Job drawing, mm, ordinate dimensions from the low corner. One solid piece. A direction names the side the tool comes from. Round coordinates to 2 decimals unless told otherwise and drop trailing zeros. Write each loop counter-clockwise with the first axis right and the second up, starting at its lowest first coordinate (ties: lowest second). Pieces come first, ordered by that corner, then holes.
1) Pull direction X, two halves, no side cores. Call the marked faces 1, 2 and 3: +X half, -X half, draft (parallel to the pull), parting line (faces both ways), or undercut.
2) Saw through at B-B (z = 15.5). Write the cut outline in (x, y).
3) Flat gauge pins, fed straight in: pin 1 (2 mm diameter, centred on y = 10, z = 14.5, fed in from +X); pin 2 (6.5 mm diameter, centred on x = 84, y = 5, fed in from -Z); pin 3 (5 mm diameter, centred on x = 31, y = 1.5, fed in from +Z). Where does each tip first touch, or does it go through?
4) Saw through at C-C (y = 5.25). Write the cut outline in (x, z), plus the area to 3 significant figures.
5) Saw through at A-A (z = 19.25). State how many separate pieces and enclosed holes the cut face has, plus the area to 3 significant figures.
6) Wall check: probe 1 along X at (y, z) = (1.5, 16); probe 2 along Z at (x, y) = (33, 8); probe 3 along Y at (x, z) = (4, 19.25). Give the ranges that are in metal, low to high.
7) Which spindle directions (+Z, -Z, +X, -X, +Y, -Y) get a long thin tool onto all of the face, cutting with end or side? Do the marked faces 4, 5 and 6. Say none if no direction does.
8) Saw through at D-D (x = 4). Write the cut outline in (y, z), plus the area to 3 significant figures.
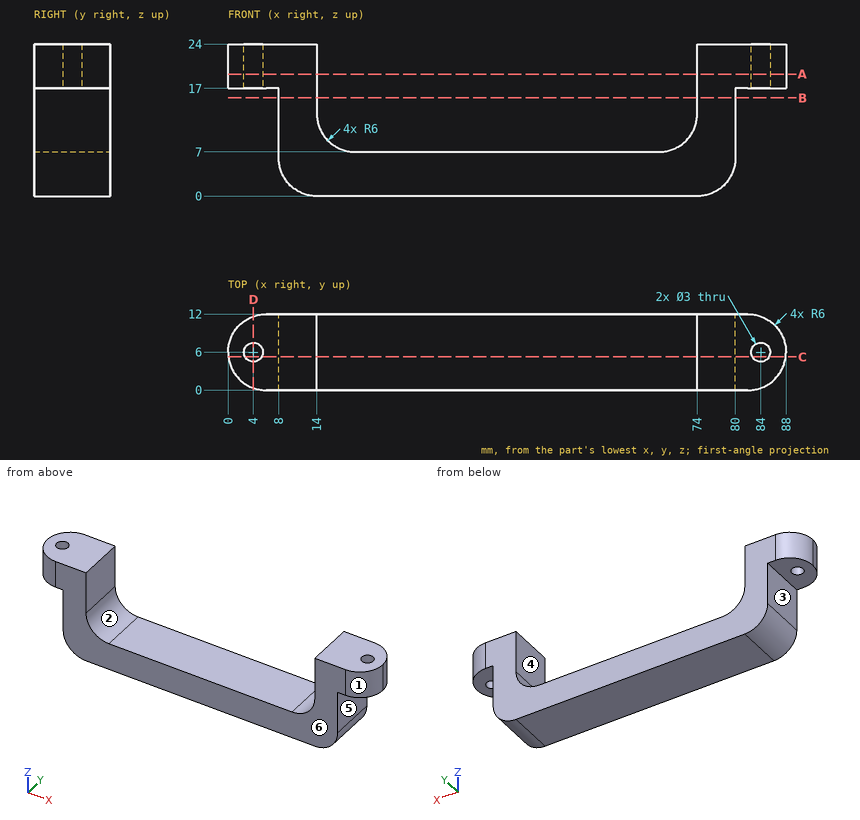
Evaluation:
1. face 1: +X half
1. face 2: undercut
1. face 3: -X half
2. outline: (8, 0) - (14, 0) - (14, 12) - (8, 12) - close; (74, 0) - (80, 0) - (80, 12) - (74, 12) - close
3. pin 1: stops at x = 80
3. pin 2: stops at z = 17
3. pin 3: stops at z = 7
4. outline: (0.05, 17) - (2.7, 17) - (2.7, 24) - (0.05, 24) - close; (5.3, 17) - (8, 17) - (8, 6) arc R6 ccw to (14, 0) - (74, 0) arc R6 ccw to (80, 6) - (80, 17) - (82.7, 17) - (82.7, 24) - (74, 24) - (74, 13) arc R6 cw to (68, 7) - (20, 7) arc R6 cw to (14, 13) - (14, 24) - (5.3, 24) - close; (85.3, 17) - (87.95, 17) - (87.95, 24) - (85.3, 24) - close
4. area: 783 mm2
5. separate pieces: 2
5. enclosed holes: 2
5. area: 291 mm2
6. probe 1: x = 8 to 14, 74 to 80
6. probe 2: z = 0 to 7
6. probe 3: y = 0.34 to 4.5, 7.5 to 11.66
7. face 4: +Z, +Y, -Y
7. face 5: -Z, +X, +Y, -Y
7. face 6: +Z, -Z, +X, -X, -Y
8. outline: (0.34, 17) - (4.5, 17) - (4.5, 24) - (0.34, 24) - close; (7.5, 17) - (11.66, 17) - (11.66, 24) - (7.5, 24) - close
8. area: 58.2 mm2
